```python
from build123d import *

# Parameters (mm, degrees)
F1_DEPTH = 203.2
F2_R     = 1
F3_W     = 94
F3_H     = 60.048782
F4_DEPTH = 300


with BuildPart() as f1:
    # F0 (on Top) → F1 (new body)
    with BuildSketch(Plane.XY):
        Polygon((-68.026056, 0), (-258.026056, 0), (-258.026056, 95), (-263.026056, 95), (-263.026056, -5), (-63.026056, -5), (-63.026056, 95), (-68.026056, 95), align=None)
    extrude(amount=F1_DEPTH)

    # F2
    f2_edges = [f1.edges().sort_by_distance(p)[0] for p in [
        (-63.026056, 95, 101.6),
        (-68.026056, 95, 101.6),
        (-258.026056, 95, 101.6),
        (-263.026056, 95, 101.6),
    ]]
    fillet(f2_edges, radius=F2_R)

    # F3 (on face) → F4 (cut)
    with BuildSketch(Plane.YZ.offset(-63.026056)):
        with Locations((47, 103.279952)):
            Rectangle(F3_W, F3_H)
    extrude(amount=-F4_DEPTH, mode=Mode.SUBTRACT)


solid = f1.part
```
Part model, mm, in its own coordinate system. A direction names the side the tool comes from. Round coordinates to 2 decimals unless told otherwise and drop trailing zeros. Write each loop counter-clockwise with the first axis right and the second up, starting at its lowest first coordinate (ties: lowest second). Pieces come first, ordered by that corner, then holes. Notation, with made-up numbers: (38.5, 13) -> (87.5, 13) arc R6 cw to (87.5, 19) -> close; hole circle Ø4 at (57.5, -27). An arc over 180 degrees is marked (long way). Return JSON: item names as keys, results as strings. Group by question number.
Q1. Which spindle directions (+Z, -Z, +X, -X, +Y, -Y) get a long thin tool onto all of the face, cutting with end or side? Do faces 1 (the flat face through (-164, -5, 100)), 2 (the flat face through (-68.026, 48, 36)), 3 (the flat face through (-260, 94, 103)). Say none if no direction does.
Q2. Saw through at C-C on z = 177.5. Write the cut outline in (x, y).
Q3. Pin check, flat tip, straight feed: pin 1 (1.5 mm diameter, centred on x = -66, y = 49.5, fed in from -Z). Stop position of the tip, or through.
Q4. Saw through at D-D on x = -194. Write the cut outline in (y, z).
Q5. Probe L1, parallel to X at y = 54, z = 156.5; L2, parallel to Y at x = -79, z = 85.5. List the from-to ranges inside material, lowest first. Write a range as [from, to].
Q6. Mould opens along X. For faces 4 (the flat face through (-263.026, 45, 55)), 5 (the flat face through (-68.026, 48, 168)), 6 (the flat face through (-63.026, -0.2, 100.2)) say: pulls with the +X half, pulls with the -X half, needs draft (parallel to the pull), parting line crosses it, or undercut.
Q7. Saw through at B-B on z = 113.5. Write the cut outline in (x, y), plus the area to 3 significant figures.
Q8. Saw through at A-A on y = 18.5. Write the cut outline in (x, z).
Answer:
{
 "1": {"face 1": "+Z, -Z, +X, -X, -Y", "face 2": "+Z, -Z, +Y", "face 3": "+X, -X"},
 "2": {"outline": "(-263.03, -5) -> (-63.03, -5) -> (-63.03, 94) arc R1 ccw to (-64.03, 95) -> (-67.03, 95) arc R1 ccw to (-68.03, 94) -> (-68.03, 0) -> (-258.03, 0) -> (-258.03, 94) arc R1 ccw to (-259.03, 95) -> (-262.03, 95) arc R1 ccw to (-263.03, 94) -> close"},
 "3": {"pin 1": "z = 0"},
 "4": {"outline": "(-5, 0) -> (0, 0) -> (0, 203.2) -> (-5, 203.2) -> close"},
 "5": {"L1": "[-263.03, -258.03], [-68.03, -63.03]", "L2": "[-5, 0]"},
 "6": {"face 4": "pulls with the -X half", "face 5": "undercut", "face 6": "pulls with the +X half"},
 "7": {"outline": "(-263.03, -5) -> (-63.03, -5) -> (-63.03, 0) -> (-263.03, 0) -> close; (-263.03, 94) -> (-258.03, 94) arc R1 ccw to (-259.03, 95) -> (-262.03, 95) arc R1 ccw to start; (-68.03, 94) -> (-63.03, 94) arc R1 ccw to (-64.03, 95) -> (-67.03, 95) arc R1 ccw to start", "area": "1,010 mm2"},
 "8": {"outline": "(-263.03, 0) -> (-258.03, 0) -> (-258.03, 73.26) -> (-263.03, 73.26) -> close; (-263.03, 133.3) -> (-258.03, 133.3) -> (-258.03, 203.2) -> (-263.03, 203.2) -> close; (-68.03, 0) -> (-63.03, 0) -> (-63.03, 73.26) -> (-68.03, 73.26) -> close; (-68.03, 133.3) -> (-63.03, 133.3) -> (-63.03, 203.2) -> (-68.03, 203.2) -> close"}
}
